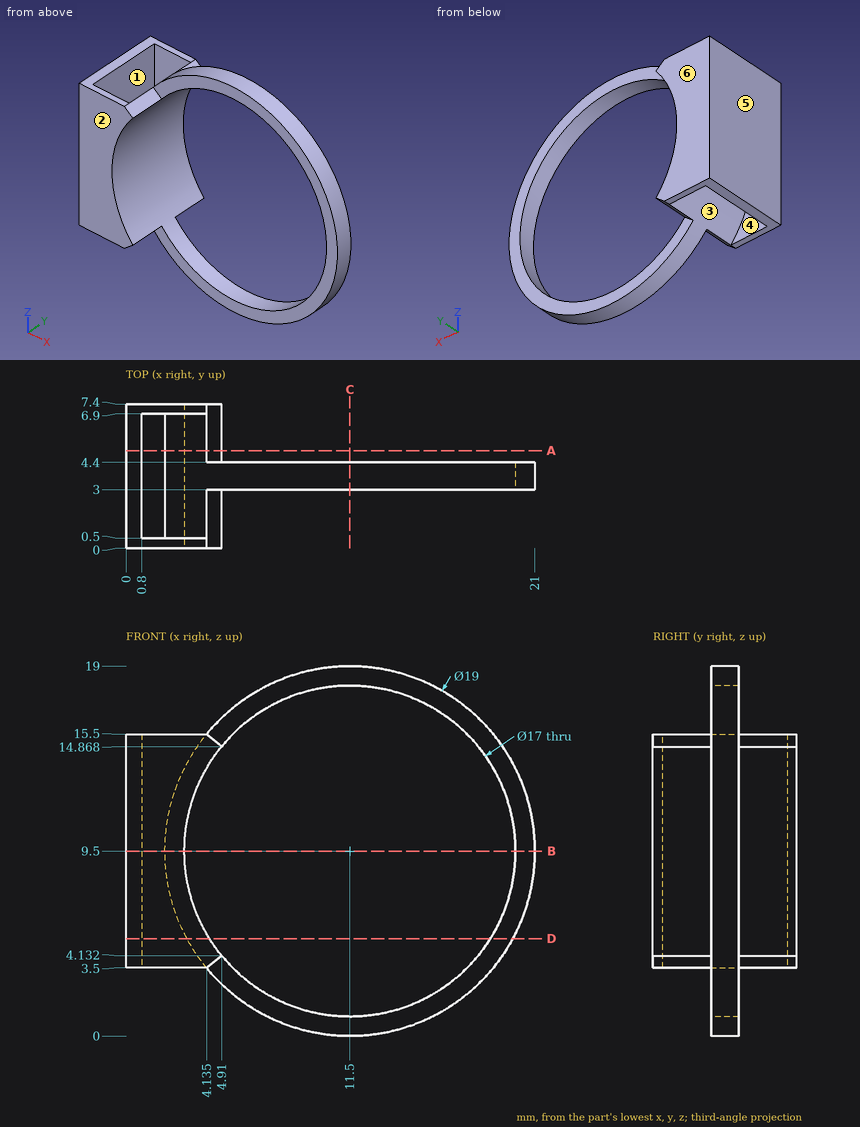
Print and shaded views of the part. All mm, measured from the part's lowest x, y and z. A direction names the side the tool comes from. Coordinates: 2 decimals unless noted, no trailing zeros. Loops run counter-clockwise (first coordinate to the right, second up) from the corner with the lowest first, then second, coordinate; pieces in that order, holes last. Notation, with made-up numbers: (40.25, 87.5) -> (66.25, 87.5) arc R26 ccw to (66.25, 122.5) -> close; hole circle Ø4 at (4.25, -24.75). An arc over 180 degrees is marked (long way). Use a Markdown table: item, result. Add a question column.
Item 1: Probe probe 1 along X at (y, z) = (4.5, 9.5); probe 2 along X at (y, z) = (4, 6.25) (1 decimal); probe 3 along Y at (x, z) = (1, 4.5). List the from-to ranges inside material, lowest first.
Item 2: Band-saw the part on A-A on y = 5. Write the cut outline in (x, z) (1 decimal).
Item 3: Which spindle directions (+Z, -Z, +X, -X, +Y, -Y) get a long thin tool onto all of the face, cutting with end or side? Do the marked faces 1, 2 and 3. Say none if no direction does.
Item 4: Flat gauge pins, fed straight in: P1, Ø3, axis at x = 17, z = 15, coming from the -Y side; P2, Ø1.5, axis at x = 6, y = 2, coming from the +Z side; P3, Ø1, axis at y = 1.5, z = 3.5, coming from the +X side; P4, Ø2, axis at x = 1.5, y = 2.5, coming from the -Z side. Where does each tip first touch, or does it go through?
Item 5: Band-saw the part on B-B on z = 9.5. Write the cut outline in (x, y).
Item 6: Pull direction X, two halves, no side cores. Call the marked faces 4, 5 and 6: +X half, -X half, draft (parallel to the pull), parting line (faces both ways), or undercut.
Item 7: Band-saw the part on D-D on z = 5. Write the cut outline in (x, y).
Item 8: Band-saw the part on C-C on x = 11.5. Write the cut outline in (y, z).
Geometry says:
| question | item | result |
|---|---|---|
| 1 | probe 1 | 0 to 0.8, 2 to 3 |
| 1 | probe 2 | 0 to 0.8, 2.6 to 3.6, 19.4 to 20.4 |
| 1 | probe 3 | 0 to 0.5, 6.9 to 7.4 |
| 2 | outline | (0, 3.5) -> (0.8, 3.5) -> (0.8, 15.5) -> (0, 15.5) -> close; (4.1, 3.5) -> (4.9, 4.1) arc R8.5 cw to (4.9, 14.9) -> (4.1, 15.5) arc R9.5 ccw to start |
| 3 | face 1 | +Z, -Z |
| 3 | face 2 | +Z, -Z, +X, -X, -Y |
| 3 | face 3 | none |
| 4 | P1 | y = 3 |
| 4 | P2 | through |
| 4 | P3 | x = 4.75 |
| 4 | P4 | z = 3.5 |
| 5 | outline | (0, 0) -> (3, 0) -> (3, 7.4) -> (0, 7.4) -> close; (20, 3) -> (21, 3) -> (21, 4.4) -> (20, 4.4) -> close; hole (0.8, 0.5) -> (2, 0.5) -> (2, 6.9) -> (0.8, 6.9) -> close |
| 6 | face 4 | undercut |
| 6 | face 5 | -X half |
| 6 | face 6 | draft |
| 7 | outline | (0, 0) -> (4.29, 0) -> (4.29, 7.4) -> (0, 7.4) -> close; (18.71, 3) -> (19.87, 3) -> (19.87, 4.4) -> (18.71, 4.4) -> close; hole (0.8, 0.5) -> (3.13, 0.5) -> (3.13, 6.9) -> (0.8, 6.9) -> close |
| 8 | outline | (3, 0) -> (4.4, 0) -> (4.4, 1) -> (3, 1) -> close; (3, 18) -> (4.4, 18) -> (4.4, 19) -> (3, 19) -> close |
